```python
from build123d import *

# Parameters (mm, degrees)
SKETCH_1_W               = 80
SKETCH_1_H               = 50
EXTRUDE_1_DEPTH          = 32
CUT_EXTRUDE_1_DEPTH      = 72.582120673
CUT_EXTRUDE_1_DEPTH_BACK = 72.582120673
SKETCH_2_R               = 7.5
HOLE_WIZARD_M5_1_D       = 4.2
HOLE_WIZARD_M5_1_DEPTH   = 11.1381927
HOLE_WIZARD_M5_1_TIP     = 1.2618073
HOLE_WIZARD_M4_1_D       = 3.3
HOLE_WIZARD_M4_1_DEPTH   = 9.108579979
HOLE_WIZARD_M4_1_TIP     = 0.991420021


with BuildPart() as part:
    # 草图1 → 凸台-拉伸1 (new body)
    with BuildSketch(Plane(origin=(0, 0, 0), x_dir=(1, 0, 0), z_dir=(0, 1, 0))):
        Rectangle(SKETCH_1_W, SKETCH_1_H)
    extrude(amount=EXTRUDE_1_DEPTH)

    # 草图2 → 切除-拉伸1 (cut, two sides: drawn at the far end of the back side and taken through both)
    with BuildSketch(Plane.XY.offset(25).offset(-CUT_EXTRUDE_1_DEPTH_BACK)):
        with Locations((0, 19)):
            Circle(SKETCH_2_R)
    extrude(amount=CUT_EXTRUDE_1_DEPTH + CUT_EXTRUDE_1_DEPTH_BACK, mode=Mode.SUBTRACT)

    # M5 螺纹孔1
    with Locations(Plane(origin=(0, 32, 0), x_dir=(1, 0, 0), z_dir=(0, 1, 0))):
        with Locations((-30, 20), (30, 20), (30, -20), (-30, -20)):
            Hole(HOLE_WIZARD_M5_1_D / 2, depth=HOLE_WIZARD_M5_1_DEPTH)
            with Locations((0, 0, -(HOLE_WIZARD_M5_1_DEPTH + HOLE_WIZARD_M5_1_TIP / 2))):  # 118° drill point
                Cone(0, HOLE_WIZARD_M5_1_D / 2, HOLE_WIZARD_M5_1_TIP, mode=Mode.SUBTRACT)

    # M4 螺纹孔1
    with Locations(Plane.ZY.offset(40)):
        with Locations((-15, 27), (15, 27)):
            Hole(HOLE_WIZARD_M4_1_D / 2, depth=HOLE_WIZARD_M4_1_DEPTH)
            with Locations((0, 0, -(HOLE_WIZARD_M4_1_DEPTH + HOLE_WIZARD_M4_1_TIP / 2))):  # 118° drill point
                Cone(0, HOLE_WIZARD_M4_1_D / 2, HOLE_WIZARD_M4_1_TIP, mode=Mode.SUBTRACT)


solid = part.part
```
Model file for the job. Use its own axes, mm. A direction names the side the tool comes from. Coordinates: 2 decimals unless noted, no trailing zeros. Loops run counter-clockwise (first coordinate to the right, second up) from the corner with the lowest first, then second, coordinate; pieces in that order, holes last. Notation, with made-up numbers: M -7.5,-2.75 L 11.5,-2.75 A11 cw 11.5,15.25 Z; hole C 60.5,0.25 d10. An arc over 180 degrees is marked long. Use CSV: the item, a comma, the result in double quotes. Start each with the question number.
1. Band-saw the part on B-B, the plane y = 13. List the corners of the cut face in (x, z), then the cut area to 3 significant figures.
2. Band-saw the part on A-A, the plane x = 0. List the corners of the cut face in (y, z).
3. Two-plate mould, pull along X, no slides. Class faces 4 (the flat face through (-40, 16, 0)), 5 (the conical face through (29.73, 19.82, 19.75)), 6 (the flat face through (-1, 9, -25)): pulls with the +X half, pulls with the -X half, needs draft (parallel to the pull), parting line crosses it, or undercut.
4. Probe probe 1 along X at (y, z) = (29.5, 20); probe 2 along Z at (x, y) = (-30, 29.5); probe 3 along Y at (x, z) = (-34, 15). List the from-to ranges inside material, lowest first. Write a range as [from, to].
5. Flat gauge pins, fed straight in: pin 1 (6.5 mm diameter, centred on x = -30, z = -20, fed in from +Y); pin 2 (3.5 mm diameter, centred on x = 30, z = 20, fed in from +Y). Where does each tip first touch, or does it go through?
6. Tool access for faces 1 (the flat face through (-1, 0, 0)), 2 (the cylindrical face through (-35.38, 28.39, 14.11)), 3 (the cylindrical face through (31.548, 26.353, -21.419)): list every direction of +Z, -Z, +X, -X, +Y, -Y with a clear straight run to the whole face (end or side of a thin tool).
7. Band-saw the part on C-C, the plane z = 0. List the corners of the cut face in (x, y).
Entries:
1,outline,"M -40,-25 L -4.5,-25 L -4.5,25 L -40,25 Z; M 4.5,-25 L 40,-25 L 40,25 L 4.5,25 Z"
1,area,"3,550 mm2"
2,outline,"M 0,-25 L 11.5,-25 L 11.5,25 L 0,25 Z; M 26.5,-25 L 32,-25 L 32,25 L 26.5,25 Z"
3,face 4,"pulls with the -X half"
3,face 5,"undercut"
3,face 6,"needs draft"
4,probe 1,"x = [-40, -32.1], [-27.9, 27.9], [32.1, 40]"
4,probe 2,"z = [-25, -22.1], [-17.9, 17.9], [22.1, 25]"
4,probe 3,"y = [0, 25.35], [28.65, 32]"
5,pin 1,"stops at y = 32"
5,pin 2,"stops at y = 20.65"
6,face 1,"+Z, -Z, +X, -X, -Y"
6,face 2,"-X"
6,face 3,"+Y"
7,outline,"M -40,0 L 40,0 L 40,32 L -40,32 Z; hole C 0,19 d15"
